from build123d import *

# Parameters (mm, degrees)
SKETCH2_W                = 21.717
SKETCH2_H                = 60.706
SKETCH2_R                = 3.175
SKETCH2_R_2              = 1.778
BOSS_EXTRUDE1_DEPTH      = 2.54
SKETCH3_W                = 21.717
SKETCH3_H                = 2.54
BOSS_EXTRUDE2_DEPTH      = 12.7
BOSS_EXTRUDE3_DEPTH      = 0.381
BOSS_EXTRUDE3_DEPTH_BACK = 0.381
SKETCH6_R                = 0.635
CUT_EXTRUDE1_DEPTH       = 62.101949054
FILLET1_R                = 5.08
FILLET2_R                = 1.27


with BuildPart() as part:
    # Sketch2 → Boss-Extrude1 (new body)
    with BuildSketch(Plane.XY):
        with Locations((0, -24.003)):
            Rectangle(SKETCH2_W, SKETCH2_H)
        Circle(SKETCH2_R, mode=Mode.SUBTRACT)
        with Locations((6.096, 0)):
            Circle(SKETCH2_R_2, mode=Mode.SUBTRACT)
        with Locations((-6.096, 0)):
            Circle(SKETCH2_R_2, mode=Mode.SUBTRACT)
    extrude(amount=BOSS_EXTRUDE1_DEPTH)

    # Sketch3 → Boss-Extrude2 (add)
    with BuildSketch(Plane.XY.offset(2.54)):
        with Locations((0, -53.086)):
            Rectangle(SKETCH3_W, SKETCH3_H)
    extrude(amount=BOSS_EXTRUDE2_DEPTH)

    # Sketch5 → Boss-Extrude3 (add, two sides: drawn at the far end of the back side and taken through both)
    with BuildSketch(Plane.ZY.offset(-BOSS_EXTRUDE3_DEPTH_BACK)):
        Polygon((15.24, -51.816), (2.54, -51.816), (2.54, -39.116), align=None)
    extrude(amount=BOSS_EXTRUDE3_DEPTH + BOSS_EXTRUDE3_DEPTH_BACK)

    # Sketch6 → Cut-Extrude1 (cut, through all)
    with BuildSketch(Plane(origin=(0, -51.816, 0), x_dir=(1, 0, 0), z_dir=(0, 1, 0))):
        with Locations(Location((-6.35, -5.715, 0), (0, 0, 270))):
            Circle(SKETCH6_R)
        with Locations(Location((6.35, -5.715, 0), (0, 0, 270))):
            Circle(SKETCH6_R)
        with Locations(Location((6.35, -12.065, 0), (0, 0, 270))):
            Circle(SKETCH6_R)
        with Locations(Location((-6.35, -12.065, 0), (0, 0, 270))):
            Circle(SKETCH6_R)
    extrude(amount=-CUT_EXTRUDE1_DEPTH, mode=Mode.SUBTRACT)

    # Fillet1
    fillet1_edges = [part.edges().sort_by_distance(p)[0] for p in [
        (10.8585, 6.35, 1.27),
        (-10.8585, 6.35, 1.27),
    ]]
    fillet(fillet1_edges, radius=FILLET1_R)

    # Fillet2
    # the kernel refuses this fillet: 1.27 mm, written as the material it adds along each edge
    with BuildSketch(Plane(origin=(0.381, -51.816, 2.54), x_dir=(1, 0, 0), z_dir=(0, 1, 0))) as fillet2_piece_1_section:
        with BuildLine():
            CenterArc((FILLET2_R, -FILLET2_R), FILLET2_R, 90, 90)
            Line((0, -FILLET2_R), (-FILLET2_R * 0.02, -FILLET2_R))
            Line((-FILLET2_R * 0.02, -FILLET2_R), (-FILLET2_R * 0.02, FILLET2_R * 0.02))
            Line((-FILLET2_R * 0.02, FILLET2_R * 0.02), (FILLET2_R, FILLET2_R * 0.02))
            Line((FILLET2_R, FILLET2_R * 0.02), (FILLET2_R, 0))
        make_face()
    fillet2_piece_1 = extrude(amount=15.875, mode=Mode.PRIVATE)
    fillet2_piece_1 = split(fillet2_piece_1, bisect_by=Plane(origin=(0.67208957, -42.502111902, 5.926111902), z_dir=(0, -0.7071067811865475, -0.7071067811865477)), keep=Keep.TOP, mode=Mode.PRIVATE)
    add(fillet2_piece_1)
    with BuildSketch(Plane(origin=(-0.381, -51.816, 2.54), x_dir=(-1, 0, 0), z_dir=(0, 1, 0))) as fillet2_piece_2_section:
        with BuildLine():
            CenterArc((FILLET2_R, FILLET2_R), FILLET2_R, 180, 90)
            Line((0, FILLET2_R), (-FILLET2_R * 0.02, FILLET2_R))
            Line((-FILLET2_R * 0.02, FILLET2_R), (-FILLET2_R * 0.02, -FILLET2_R * 0.02))
            Line((-FILLET2_R * 0.02, -FILLET2_R * 0.02), (FILLET2_R, -FILLET2_R * 0.02))
            Line((FILLET2_R, -FILLET2_R * 0.02), (FILLET2_R, 0))
        make_face()
    fillet2_piece_2 = extrude(amount=15.875, mode=Mode.PRIVATE)
    fillet2_piece_2 = split(fillet2_piece_2, bisect_by=Plane(origin=(-0.67208957, -42.502111902, 5.926111902), z_dir=(0, -0.7071067811865475, -0.7071067811865477)), keep=Keep.TOP, mode=Mode.PRIVATE)
    add(fillet2_piece_2)
    with BuildSketch(Plane(origin=(-0.381, -51.816, 15.24), x_dir=(0, 1, 0), z_dir=(0, 0, -1))) as fillet2_piece_3_section:
        with BuildLine():
            CenterArc((FILLET2_R, -FILLET2_R), FILLET2_R, 90, 90)
            Line((0, -FILLET2_R), (-FILLET2_R * 0.02, -FILLET2_R))
            Line((-FILLET2_R * 0.02, -FILLET2_R), (-FILLET2_R * 0.02, FILLET2_R * 0.02))
            Line((-FILLET2_R * 0.02, FILLET2_R * 0.02), (FILLET2_R, FILLET2_R * 0.02))
            Line((FILLET2_R, FILLET2_R * 0.02), (FILLET2_R, 0))
        make_face()
    fillet2_piece_3 = extrude(amount=12.7, mode=Mode.PRIVATE)
    fillet2_piece_3 = split(fillet2_piece_3, bisect_by=Plane(origin=(-0.672062457, -48.429609874, 11.853609874), z_dir=(0, -0.7071067811865475, -0.7071067811865477)), keep=Keep.TOP, mode=Mode.PRIVATE)
    add(fillet2_piece_3)
    with BuildSketch(Plane(origin=(0.381, -51.816, 15.24), x_dir=(1, 0, 0), z_dir=(0, 0, -1))) as fillet2_piece_4_section:
        with BuildLine():
            CenterArc((FILLET2_R, -FILLET2_R), FILLET2_R, 90, 90)
            Line((0, -FILLET2_R), (-FILLET2_R * 0.02, -FILLET2_R))
            Line((-FILLET2_R * 0.02, -FILLET2_R), (-FILLET2_R * 0.02, FILLET2_R * 0.02))
            Line((-FILLET2_R * 0.02, FILLET2_R * 0.02), (FILLET2_R, FILLET2_R * 0.02))
            Line((FILLET2_R, FILLET2_R * 0.02), (FILLET2_R, 0))
        make_face()
    fillet2_piece_4 = extrude(amount=12.7, mode=Mode.PRIVATE)
    fillet2_piece_4 = split(fillet2_piece_4, bisect_by=Plane(origin=(0.672062457, -48.429609874, 11.853609874), z_dir=(0, -0.7071067811865475, -0.7071067811865477)), keep=Keep.TOP, mode=Mode.PRIVATE)
    add(fillet2_piece_4)
    with BuildSketch(Plane(origin=(0.381, -39.116, 2.54), x_dir=(0, 1, 0), z_dir=(-1, 0, 0))) as fillet2_piece_5:
        with BuildLine():
            CenterArc((FILLET2_R * 0.414213562373, -FILLET2_R), FILLET2_R, 90, 45)
            Line((-FILLET2_R * 0.292893218813, -FILLET2_R * 0.292893218813), (-FILLET2_R * 0.307035354437, -FILLET2_R * 0.27875108319))
            Line((-FILLET2_R * 0.307035354437, -FILLET2_R * 0.27875108319), (-FILLET2_R * 0.00828427124746, FILLET2_R * 0.02))
            Line((-FILLET2_R * 0.00828427124746, FILLET2_R * 0.02), (FILLET2_R * 0.414213562373, FILLET2_R * 0.02))
            Line((FILLET2_R * 0.414213562373, FILLET2_R * 0.02), (FILLET2_R * 0.414213562373, 0))
        make_face()
    extrude(amount=0.762)
    with BuildSketch(Plane(origin=(0.381, -54.991, 2.54), x_dir=(1, 0, 0), z_dir=(0, 1, 0))) as fillet2_piece_6a_section:
        with BuildLine():
            CenterArc((FILLET2_R, -FILLET2_R), FILLET2_R, 90, 90)
            Line((0, -FILLET2_R), (-FILLET2_R * 0.02, -FILLET2_R))
            Line((-FILLET2_R * 0.02, -FILLET2_R), (-FILLET2_R * 0.02, FILLET2_R * 0.02))
            Line((-FILLET2_R * 0.02, FILLET2_R * 0.02), (FILLET2_R, FILLET2_R * 0.02))
            Line((FILLET2_R, FILLET2_R * 0.02), (FILLET2_R, 0))
        make_face()
    fillet2_piece_6a = extrude(amount=19.05, mode=Mode.PRIVATE)
    fillet2_piece_6a = split(fillet2_piece_6a, bisect_by=Plane(origin=(0.668521795, -51.816, 2.827521795), z_dir=(0, -1, 0)), keep=Keep.TOP, mode=Mode.PRIVATE)
    with BuildSketch(Plane(origin=(0.381, -51.816, 15.24), x_dir=(1, 0, 0), z_dir=(0, 0, -1))) as fillet2_piece_6b_section:
        with BuildLine():
            CenterArc((FILLET2_R, -FILLET2_R), FILLET2_R, 90, 90)
            Line((0, -FILLET2_R), (-FILLET2_R * 0.02, -FILLET2_R))
            Line((-FILLET2_R * 0.02, -FILLET2_R), (-FILLET2_R * 0.02, FILLET2_R * 0.02))
            Line((-FILLET2_R * 0.02, FILLET2_R * 0.02), (FILLET2_R, FILLET2_R * 0.02))
            Line((FILLET2_R, FILLET2_R * 0.02), (FILLET2_R, 0))
        make_face()
    fillet2_piece_6b = extrude(amount=15.875, mode=Mode.PRIVATE)
    fillet2_piece_6b = split(fillet2_piece_6b, bisect_by=Plane(origin=(0.668521795, -51.528478205, 2.54), z_dir=(0, 0, -1)), keep=Keep.TOP, mode=Mode.PRIVATE)
    fillet2_piece_6 = fillet2_piece_6a & fillet2_piece_6b
    add(fillet2_piece_6)
    with BuildSketch(Plane(origin=(0.381, -51.816, 2.54), x_dir=(1, 0, 0), z_dir=(0, 1, 0))) as fillet2_piece_7a_section:
        with BuildLine():
            CenterArc((FILLET2_R, -FILLET2_R), FILLET2_R, 90, 90)
            Line((0, -FILLET2_R), (-FILLET2_R * 0.02, -FILLET2_R))
            Line((-FILLET2_R * 0.02, -FILLET2_R), (-FILLET2_R * 0.02, FILLET2_R * 0.02))
            Line((-FILLET2_R * 0.02, FILLET2_R * 0.02), (FILLET2_R, FILLET2_R * 0.02))
            Line((FILLET2_R, FILLET2_R * 0.02), (FILLET2_R, 0))
        make_face()
    fillet2_piece_7a = extrude(amount=15.875, mode=Mode.PRIVATE)
    fillet2_piece_7a = split(fillet2_piece_7a, bisect_by=Plane(origin=(0.655732005, -38.554128536, 1.978128536), z_dir=(0, 0.7071067811865475, 0.7071067811865477)), keep=Keep.TOP, mode=Mode.PRIVATE)
    with BuildSketch(Plane(origin=(1.696128061, -39.116, 2.54), x_dir=(0, 1, 0), z_dir=(-1, 0, 0))) as fillet2_piece_7b_section:
        with BuildLine():
            CenterArc((FILLET2_R * 0.414213562373, -FILLET2_R), FILLET2_R, 90, 45)
            Line((-FILLET2_R * 0.292893218813, -FILLET2_R * 0.292893218813), (-FILLET2_R * 0.307035354437, -FILLET2_R * 0.27875108319))
            Line((-FILLET2_R * 0.307035354437, -FILLET2_R * 0.27875108319), (-FILLET2_R * 0.00828427124746, FILLET2_R * 0.02))
            Line((-FILLET2_R * 0.00828427124746, FILLET2_R * 0.02), (FILLET2_R * 0.414213562373, FILLET2_R * 0.02))
            Line((FILLET2_R * 0.414213562373, FILLET2_R * 0.02), (FILLET2_R * 0.414213562373, 0))
        make_face()
    fillet2_piece_7b = extrude(amount=2.077128061, mode=Mode.PRIVATE)
    fillet2_piece_7b = split(fillet2_piece_7b, bisect_by=Plane(origin=(0.381, -39.083484699, 2.618498881), z_dir=(1, 0, 0)), keep=Keep.TOP, mode=Mode.PRIVATE)
    fillet2_piece_7 = fillet2_piece_7a & fillet2_piece_7b
    add(fillet2_piece_7)
    with BuildSketch(Plane(origin=(-0.381, -54.991, 2.54), x_dir=(-1, 0, 0), z_dir=(0, 1, 0))) as fillet2_piece_8a_section:
        with BuildLine():
            CenterArc((FILLET2_R, FILLET2_R), FILLET2_R, 180, 90)
            Line((0, FILLET2_R), (-FILLET2_R * 0.02, FILLET2_R))
            Line((-FILLET2_R * 0.02, FILLET2_R), (-FILLET2_R * 0.02, -FILLET2_R * 0.02))
            Line((-FILLET2_R * 0.02, -FILLET2_R * 0.02), (FILLET2_R, -FILLET2_R * 0.02))
            Line((FILLET2_R, -FILLET2_R * 0.02), (FILLET2_R, 0))
        make_face()
    fillet2_piece_8a = extrude(amount=19.05, mode=Mode.PRIVATE)
    fillet2_piece_8a = split(fillet2_piece_8a, bisect_by=Plane(origin=(-0.668521795, -51.816, 2.827521795), z_dir=(0, -1, 0)), keep=Keep.TOP, mode=Mode.PRIVATE)
    with BuildSketch(Plane(origin=(-0.381, -51.816, 15.24), x_dir=(0, 1, 0), z_dir=(0, 0, -1))) as fillet2_piece_8b_section:
        with BuildLine():
            CenterArc((FILLET2_R, -FILLET2_R), FILLET2_R, 90, 90)
            Line((0, -FILLET2_R), (-FILLET2_R * 0.02, -FILLET2_R))
            Line((-FILLET2_R * 0.02, -FILLET2_R), (-FILLET2_R * 0.02, FILLET2_R * 0.02))
            Line((-FILLET2_R * 0.02, FILLET2_R * 0.02), (FILLET2_R, FILLET2_R * 0.02))
            Line((FILLET2_R, FILLET2_R * 0.02), (FILLET2_R, 0))
        make_face()
    fillet2_piece_8b = extrude(amount=15.875, mode=Mode.PRIVATE)
    fillet2_piece_8b = split(fillet2_piece_8b, bisect_by=Plane(origin=(-0.668521795, -51.528478205, 2.54), z_dir=(0, 0, -1)), keep=Keep.TOP, mode=Mode.PRIVATE)
    fillet2_piece_8 = fillet2_piece_8a & fillet2_piece_8b
    add(fillet2_piece_8)
    with BuildSketch(Plane(origin=(0.381, -39.116, 2.54), x_dir=(0, 1, 0), z_dir=(-1, 0, 0))) as fillet2_piece_9a_section:
        with BuildLine():
            CenterArc((FILLET2_R * 0.414213562373, -FILLET2_R), FILLET2_R, 90, 45)
            Line((-FILLET2_R * 0.292893218813, -FILLET2_R * 0.292893218813), (-FILLET2_R * 0.307035354437, -FILLET2_R * 0.27875108319))
            Line((-FILLET2_R * 0.307035354437, -FILLET2_R * 0.27875108319), (-FILLET2_R * 0.00828427124746, FILLET2_R * 0.02))
            Line((-FILLET2_R * 0.00828427124746, FILLET2_R * 0.02), (FILLET2_R * 0.414213562373, FILLET2_R * 0.02))
            Line((FILLET2_R * 0.414213562373, FILLET2_R * 0.02), (FILLET2_R * 0.414213562373, 0))
        make_face()
    fillet2_piece_9a = extrude(amount=2.077128061, mode=Mode.PRIVATE)
    fillet2_piece_9a = split(fillet2_piece_9a, bisect_by=Plane(origin=(-0.381, -39.083484699, 2.618498881), z_dir=(-1, 0, 0)), keep=Keep.TOP, mode=Mode.PRIVATE)
    with BuildSketch(Plane(origin=(-0.381, -51.816, 2.54), x_dir=(-1, 0, 0), z_dir=(0, 1, 0))) as fillet2_piece_9b_section:
        with BuildLine():
            CenterArc((FILLET2_R, FILLET2_R), FILLET2_R, 180, 90)
            Line((0, FILLET2_R), (-FILLET2_R * 0.02, FILLET2_R))
            Line((-FILLET2_R * 0.02, FILLET2_R), (-FILLET2_R * 0.02, -FILLET2_R * 0.02))
            Line((-FILLET2_R * 0.02, -FILLET2_R * 0.02), (FILLET2_R, -FILLET2_R * 0.02))
            Line((FILLET2_R, -FILLET2_R * 0.02), (FILLET2_R, 0))
        make_face()
    fillet2_piece_9b = extrude(amount=15.875, mode=Mode.PRIVATE)
    fillet2_piece_9b = split(fillet2_piece_9b, bisect_by=Plane(origin=(-0.655732005, -38.554128536, 1.978128536), z_dir=(0, 0.7071067811865475, 0.7071067811865477)), keep=Keep.TOP, mode=Mode.PRIVATE)
    fillet2_piece_9 = fillet2_piece_9a & fillet2_piece_9b
    add(fillet2_piece_9)


solid = part.part
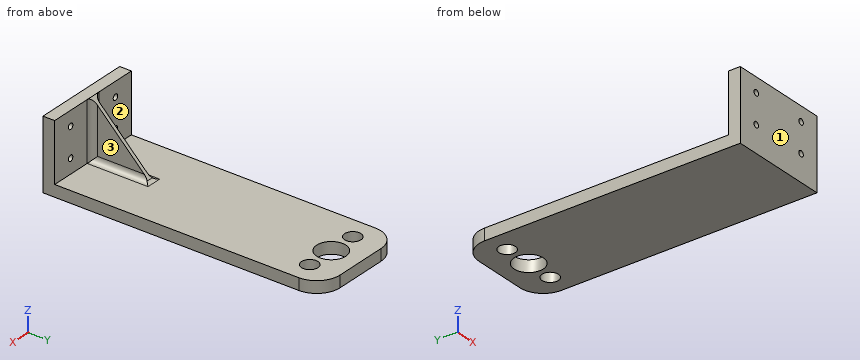
Design review of the part built by this model. Coordinates are the model's own, in mm. Face numbers are marked on the shaded views. A direction names the side the tool comes from. Coordinates: 2 decimals unless noted, no trailing zeros. Write each loop counter-clockwise with the first axis right and the second up, starting at its lowest first coordinate (ties: lowest second). Pieces come first, ordered by that corner, then holes. Notation, with made-up numbers: (10, 12) -> (29, 12) arc R5 cw to (29, 20) -> close; hole circle Ø5 at (82.5, 81.5). An arc over 180 degrees is marked (long way). Write each question's results on one line, items separated by ' | '. Start each with the question number.
(1) Take a section at B-B on x = 6.35. Write out the cut boundary in (y, z).
(2) Take a section at D-D on x = -2.5. Write out the cut boundary in (y, z), and give its area (3 significant figures).
(3) Tool access review of the marked faces 1, 2 and 3: name each direction out of +Z, -Z, +X, -X, +Y, -Y from which nothing blocks a thin tool from reaching the whole face with its end or side.
(4) Take a section at A-A on y = -2.5. Write out the cut boundary in (x, z), and give its area (3 significant figures).
(5) Clearance check with flat-ended pins moving along their axes: P1, Ø2, axis at x = 6.35, z = 12.065, coming from the -Y side; P2, Ø3, axis at x = 6.096, y = 0, coming from the +Z side; P3, Ø3, axis at x = 2.5, y = -45.5, coming from the +Z side; P4, Ø5, axis at y = -46.5, z = 8, coming from the +X side. State where each tip first meets the part, or that it passes through.
(6) Take a section at C-C on z = 10.25. Write out the cut boundary in (x, y), and give its area (3 significant figures).
(7) For line 1 along Z through (x, y) = (0.25, -27.5); line 2 along Y through (x, z) = (5.5, 12.25); line 3 along X through (y, z) = (-49.5, 10.75), list the stretches that pass through material, from the lowest coordinate up. Write a range as from..to.
Results found:
1) outline: (-54.36, 0) -> (-1.76, 0) -> (-1.76, 2.54) -> (-51.82, 2.54) -> (-51.82, 5.08) -> (-54.36, 5.08) -> close; (-54.36, 6.35) -> (-51.82, 6.35) -> (-51.82, 11.43) -> (-54.36, 11.43) -> close; (-54.36, 12.7) -> (-51.82, 12.7) -> (-51.82, 15.24) -> (-54.36, 15.24) -> close; (1.76, 0) -> (6.32, 0) -> (6.32, 2.54) -> (1.76, 2.54) -> close
2) outline: (-54.36, 0) -> (-1.96, 0) -> (-1.96, 2.54) -> (-51.82, 2.54) -> (-51.82, 15.24) -> (-54.36, 15.24) -> close; (1.96, 0) -> (6.35, 0) -> (6.35, 2.54) -> (1.96, 2.54) -> close | area: 177 mm2
3) face 1: +Z, -Z, +X, -X, -Y | face 2: +Z, -X, +Y | face 3: +Z, +X, +Y
4) outline: (-10.86, 0) -> (-1.96, 0) -> (-1.96, 2.54) -> (-10.86, 2.54) -> close; (1.96, 0) -> (10.86, 0) -> (10.86, 2.54) -> (1.96, 2.54) -> close | area: 45.2 mm2
5) P1: stops at y = -54.36 | P2: passes through | P3: stops at z = 2.72 | P4: stops at x = 0.38
6) outline: (-10.86, -54.36) -> (10.86, -54.36) -> (10.86, -51.82) -> (1.65, -51.82) arc R1.27 cw to (0.38, -50.55) -> (0.38, -46.83) -> (-0.38, -46.83) -> (-0.38, -50.55) arc R1.27 cw to (-1.65, -51.82) -> (-10.86, -51.82) -> close | area: 59.7 mm2
7) line 1: z = 0..2.54 | line 2: y = -54.36..-51.82 | line 3: x = -0.38..0.38
